CAD build for the part. Positions are in the model's coordinates, mm. A direction names the side the tool comes from. Coordinates: 2 decimals unless noted, no trailing zeros. Order: outer loops, then holes, each group sorted by start corner. A loop starts at its lowest first (then second) coordinate and runs counter-clockwise, first axis right, second up. Notation, with made-up numbers: (16.5, 40.25) - (29.5, 40.25) arc R28 ccw to (29.5, 67.25) - close; hole circle Ø9 at (31.5, 84). An arc over 180 degrees is marked (long way). Return JSON: item names as keys, results as strings.
from build123d import *

# Parameters (mm, degrees)
SKETCH1_R           = 1.25
SKETCH1_R_2         = 0.7
BOSS_EXTRUDE1_DEPTH = 12.45
DRAFT1_ANGLE        = -2
BOSS_EXTRUDE2_START = -3.175
SKETCH2_R           = 1.25
BOSS_EXTRUDE2_DEPTH = 3.175
BOSS_EXTRUDE3_START = -2.3495
SKETCH3_R           = 1.6129
SKETCH3_R_2         = 1.25
BOSS_EXTRUDE3_DEPTH = 2.3495
DRAFT2_ANGLE        = -3
CHAMFER1_SIZE       = 0.508
CHAMFER1_SIZE2      = 0.491158032
CHAMFER2_SIZE       = 0.508
CHAMFER2_SIZE2      = 0.536831287


with BuildPart() as part:
    # Sketch1 → Boss-Extrude1 (new body)
    with BuildSketch(Plane.XY):
        with Locations(Location((0, 6.009690382, 0), (0, 0, 270))):
            Circle(SKETCH1_R)
        with Locations(Location((0, 6.009690382, 0), (0, 0, 270))):
            Circle(SKETCH1_R_2, mode=Mode.SUBTRACT)
    extrude(amount=BOSS_EXTRUDE1_DEPTH)

    # Draft1
    draft1_faces = [part.faces().sort_by_distance(p)[0] for p in [
        (0, 6.709690382, 6.225),
    ]]
    draft(draft1_faces, Plane(origin=(0, 6.009690382, 0), x_dir=(-1, 0, 0), z_dir=(0, 0, -1)), DRAFT1_ANGLE)

    # Sketch2 → Boss-Extrude2 (add)
    with BuildSketch(Plane.XY.offset(12.45).offset(BOSS_EXTRUDE2_START)):
        with Locations(Location((0, 6.009690382, 0), (0, 0, 270))):
            Circle(SKETCH2_R)
    extrude(amount=BOSS_EXTRUDE2_DEPTH)

    # Sketch3 → Boss-Extrude3 (add)
    with BuildSketch(Plane.XY.offset(12.45).offset(BOSS_EXTRUDE3_START)):
        with Locations((0, 6.009690382)):
            Circle(SKETCH3_R)
        with Locations((0, 6.009690382)):
            Circle(SKETCH3_R_2, mode=Mode.SUBTRACT)
    extrude(amount=BOSS_EXTRUDE3_DEPTH)

    # Draft2
    draft2_faces = [part.faces().sort_by_distance(p)[0] for p in [
        (-1.6129, 6.009690382, 11.27525),
    ]]
    draft(draft2_faces, Plane(origin=(0, 6.009690382, 10.1005), x_dir=(-1, 0, 0), z_dir=(0, 0, -1)), DRAFT2_ANGLE)

    # Chamfer1
    chamfer1_edges = [part.edges().sort_by_distance(p)[0] for p in [
        (0, 6.709690382, 0),
    ]]
    chamfer1_side = [part.faces().sort_by_distance(p)[0] for p in [
        (0, 6.871635451, 4.6375),
    ]]
    chamfer(chamfer1_edges, length=CHAMFER1_SIZE, length2=CHAMFER1_SIZE2, reference=chamfer1_side[0])

    # Chamfer2
    chamfer2_edges = [part.edges().sort_by_distance(p)[0] for p in [
        (-1.489767923, 6.009690382, 12.45),
    ]]
    chamfer2_side = [part.faces().sort_by_distance(p)[0] for p in [
        (-1.551333961, 6.009690382, 11.27525),
    ]]
    chamfer(chamfer2_edges, length=CHAMFER2_SIZE, length2=CHAMFER2_SIZE2, reference=chamfer2_side[0])


solid = part.part
Item 1: Wall check: L1, parallel to Z at x = 0.05, y = 5.95 (3 decimals); L2, parallel to Y at x = 0.2, z = 4.25; L3, parallel to X at y = 6.2, z = 2.5. Give the ranges that are in metal, low to high. Write a range as [from, to].
Findings below:
{"L1": "z = [9.275, 12.45]", "L2": "y = [4.78, 5.19], [6.83, 7.24]", "L3": "x = [-1.24, -0.76], [0.76, 1.24]"}
Item 2: Band-saw the part on B-B, the plane z = 1.25. List the corners of the cut face in (x, y), then the cut area to 3 significant figures.
Findings below:
{"outline": "circle Ø2.5 at (0, 6.01); hole circle Ø1.49 at (0, 6.01)", "area": "3.17 mm²"}
Item 3: Which spindle directions (+Z, -Z, +X, -X, +Y, -Y) get a long thin tool onto all of the face, cutting with end or side? Do faces 4 (the cylindrical face through (0.38, 4.82, 4.98)), 5 (the conical face through (-0.333, 5.207, 4.83)). Say none if no direction does.
Findings below:
{"face 4": "-Z", "face 5": "none"}
Item 4: Band-saw the part on A-A, the plane z = 9.5. List the corners of the cut face in (x, y), then the cut area to 3 significant figures.
Findings below:
{"outline": "circle Ø2.5 at (0, 6.01)", "area": "4.91 mm²"}
Item 5: Band-saw the part on C-C, the plane z = 4.75. List the corners of the cut face in (x, y).
Findings below:
{"outline": "circle Ø2.5 at (0, 6.01); hole circle Ø1.73 at (0, 6.01)"}
Item 6: Drop flat-ended pins along their axis: P1, Ø0.6, axis at x = 0, y = 6, coming from the -Z side (3 decimals); P2, Ø1, axis at x = 0, y = 7, coming from the -Z side; P3, Ø1, axis at y = 5.5, z = 5, coming from the -X side. Give the stop position or say it passes through.
Findings below:
{"P1": "stops at z = 9.275", "P2": "stops at z = 0", "P3": "stops at x = -1.25"}
Item 7: Mould opens along Y. For faces 1 (the conical face through (0.84, 7.33, 11.01)), 2 (the flat face through (0, 6, 9.275)), 3 (the flat face through (0, 6, 12.45)) say: released by +Y, released by -Y, zero draft, split by the parting line, or undercut.
Findings below:
{"face 1": "split by the parting line", "face 2": "undercut", "face 3": "zero draft"}
